from build123d import *

# Parameters (mm, degrees)
SKETCH2_W           = 63
SKETCH2_H           = 53
BOSS_EXTRUDE1_DEPTH = 121.3
BOSS_EXTRUDE2_START = 121.3
SKETCH2_3_W         = 63
SKETCH2_3_H         = 53
BOSS_EXTRUDE2_DEPTH = 28
CHAMFER5_SIZE       = 15.5
SKETCH7_R           = 6
CUT_EXTRUDE3_DEPTH  = 5.5
FILLET5_R           = 2
SHELL2_START        = 3
SHELL2_DEPTH        = 115.3
SHELL2_START_2      = 134.895176786
SHELL2_2_DEPTH      = 11.404823214
SHELL2_START_3      = 118.3
SHELL2_3_DEPTH      = 0.6
SHELL2_START_4      = -35.5
SHELL2_4_DEPTH      = 51.5
SHELL2_START_5      = 16
SHELL2_5_DEPTH      = 8.5
SHELL2_START_6      = -25.165077586
SHELL2_6_DEPTH      = 3
SKETCH4_W           = 12
SKETCH4_H           = 115.3
CUT_EXTRUDE1_DEPTH  = 175.228269807
BOSS_EXTRUDE5_START = -3
BOSS_EXTRUDE5_DEPTH = 3
CUT_EXTRUDE2_REACH  = 168.939
SKETCH6_R           = 2.1
SKETCH8_R           = 1.45
CUT_EXTRUDE4_DEPTH  = 3
BOSS_EXTRUDE6_START = 8
SKETCH8_3_R         = 1.45
BOSS_EXTRUDE6_DEPTH = 8
CUT_EXTRUDE5_REACH  = 168.939
BOSS_EXTRUDE7_START = 3
BOSS_EXTRUDE7_DEPTH = 3
CHAMFER7_SIZE       = 3
FILLET6_R           = 5


with BuildPart() as part:
    # Sketch2 → Boss-Extrude1 (new body)
    with BuildSketch(Plane(origin=(0, 0, 0), x_dir=(1, 0, 0), z_dir=(0, 1, 0))):
        Polygon((24.5, -11), (24.5, 21), (-27.6, 21), (-27.6, 4.5), (-38.5, -11), align=None)
        with Locations((-7, -37.5)):
            Rectangle(SKETCH2_W, SKETCH2_H)
    extrude(amount=BOSS_EXTRUDE1_DEPTH)

    # Sketch2<3> → Boss-Extrude2 (add)
    with BuildSketch(Plane(origin=(0, 0, 0), x_dir=(1, 0, 0), z_dir=(0, 1, 0)).offset(BOSS_EXTRUDE2_START)):
        with Locations((-7, -37.5)):
            Rectangle(SKETCH2_3_W, SKETCH2_3_H)
    extrude(amount=BOSS_EXTRUDE2_DEPTH)

    # Chamfer5
    chamfer5_edges = [part.edges().sort_by_distance(p)[0] for p in [
        (-7, 121.3, 11),
    ]]
    chamfer(chamfer5_edges, length=CHAMFER5_SIZE)

    # Sketch7 → Cut-Extrude3 (cut)
    with BuildSketch(Plane(origin=(24.5, 0, 0), x_dir=(0, 0, -1), z_dir=(1, 0, 0))):
        with Locations((-7.675, 127.9)):
            Circle(SKETCH7_R)
    extrude(amount=-CUT_EXTRUDE3_DEPTH, mode=Mode.SUBTRACT)

    # Fillet5
    fillet5_edges = [part.edges().sort_by_distance(p)[0] for p in [
        (21.75, 133.885912692, 8.085912692),
        (21.75, 127.489087308, 1.689087308),
    ]]
    fillet(fillet5_edges, radius=FILLET5_R)

    # Shell2: read off the stored shape, not the designer's step
    # Shell2 outline → Shell2 (cut)
    with BuildSketch(Plane(origin=(0, 0, 0), x_dir=(1, 0, 0), z_dir=(0, 1, 0)).offset(SHELL2_START)):
        Polygon((-24.6, 3.550767359), (-35.5, -11.949232641), (-35.5, -61), (24.5, -61), (24.5, 18), (-24.6, 18), align=None)
    extrude(amount=SHELL2_DEPTH, mode=Mode.SUBTRACT)

    # Shell2 2 outline → Shell2 2 (cut)
    with BuildSketch(Plane(origin=(0, 0, 0), x_dir=(1, 0, 0), z_dir=(0, 1, 0)).offset(SHELL2_START_2)):
        Polygon((16, -14), (-35.5, -14), (-35.5, -61), (24.5, -61), (24.5, -14), align=None)
    extrude(amount=SHELL2_2_DEPTH, mode=Mode.SUBTRACT)

    # Shell2 3 outline → Shell2 3 (cut)
    with BuildSketch(Plane(origin=(0, 0, 0), x_dir=(1, 0, 0), z_dir=(0, 1, 0)).offset(SHELL2_START_3)):
        Polygon((16, -14), (-35.5, -14), (-35.5, -61), (24.5, -61), (24.5, -14), align=None)
    extrude(amount=SHELL2_3_DEPTH, mode=Mode.SUBTRACT)

    # Shell2 4 outline → Shell2 4 (cut)
    with BuildSketch(Plane.YZ.offset(SHELL2_START_4)):
        Polygon((134.895176786, 61), (118.9, 61), (118.9, 14), (118.3, 14), (118.3, -3.257359313), (135.557359313, 14), (134.895176786, 14), align=None)
    extrude(amount=SHELL2_4_DEPTH, mode=Mode.SUBTRACT)

    # Shell2 5 outline → Shell2 5 (cut)
    with BuildSketch(Plane.YZ.offset(SHELL2_START_5)):
        with BuildLine():
            Line((134.895176786, 61), (118.9, 61))
            Line((118.9, 61), (118.9, 14))
            Line((118.9, 14), (118.3, 14))
            Line((118.3, 14), (118.3, -3.257359313))
            Line((118.3, -3.257359313), (122.237182527, 0.679823214))
            ThreePointArc((122.237182527, 0.679823214), (121.536038969, 14.038961031), (134.895176786, 13.337817473))
            Line((134.895176786, 13.337817473), (135.557359313, 14))
            Line((135.557359313, 14), (134.895176786, 14))
            Line((134.895176786, 14), (134.895176786, 61))
        make_face()
    extrude(amount=SHELL2_5_DEPTH, mode=Mode.SUBTRACT)

    # Shell2 6 outline → Shell2 6 (add)
    with BuildSketch(Plane(origin=(0, 0, 0), x_dir=(0.5752319297142107, 0, -0.8179903587679168), z_dir=(0.8179903587679168, 0, 0.5752319297142109)).offset(SHELL2_START_6)):
        Polygon((-30.1950906, 3), (-11.246212005, 3), (-11.246212005, 118.3), (-11.604905776, 118.3), (-30.1950906, 133.506591954), align=None)
    extrude(amount=SHELL2_6_DEPTH)

    # Sketch4 → Cut-Extrude1 (cut, through all)
    with BuildSketch(Plane(origin=(24.5, 0, 0), x_dir=(0, 0, -1), z_dir=(1, 0, 0))):
        with Locations((15, 60.65)):
            Rectangle(SKETCH4_W, SKETCH4_H)
    extrude(amount=-CUT_EXTRUDE1_DEPTH, mode=Mode.SUBTRACT)

    # Sketch5 → Boss-Extrude5 (add)
    with BuildSketch(Plane(origin=(24.5, 0, 0), x_dir=(0, 0, -1), z_dir=(1, 0, 0)).offset(BOSS_EXTRUDE5_START)):
        with BuildLine():
            Line((3.257359313, 118.3), (-61, 118.3))
            Line((-61, 118.3), (-61, 146.3))
            Line((-61, 146.3), (-14, 146.3))
            Line((-14, 146.3), (-14, 135.557359313))
            Line((-14, 135.557359313), (-13.337817473, 134.895176786))
            ThreePointArc((-13.337817473, 134.895176786), (-14.038961031, 121.536038969), (-0.679823214, 122.237182527))
            Line((-0.679823214, 122.237182527), (3.257359313, 118.3))
        make_face()
    extrude(amount=BOSS_EXTRUDE5_DEPTH)

    # Cut-Extrude2: up to this face of the body (flat: up to its plane)
    cut_extrude2_end = Plane(part.part.faces().sort_by_distance((-1.55, 121.3, -12.75))[0])
    # Sketch6 → Cut-Extrude2 (cut, up to the picked face)
    with BuildSketch(Plane.XZ, mode=Mode.PRIVATE) as cut_extrude2_sk1:
        with Locations(Location((-12.5, -11.5, 0), (0, 0, 270))):
            Circle(SKETCH6_R)
    cut_extrude2_tool1 = split(extrude(cut_extrude2_sk1.sketch, amount=-CUT_EXTRUDE2_REACH, mode=Mode.PRIVATE), bisect_by=cut_extrude2_end, keep=Keep.BOTH, mode=Mode.PRIVATE)
    # Sketch6 → Cut-Extrude2 (cut, up to the picked face)
    with BuildSketch(Plane.XZ, mode=Mode.PRIVATE) as cut_extrude2_sk2:
        with Locations(Location((12.5, -11.5, 0), (0, 0, 270))):
            Circle(SKETCH6_R)
    cut_extrude2_tool2 = split(extrude(cut_extrude2_sk2.sketch, amount=-CUT_EXTRUDE2_REACH, mode=Mode.PRIVATE), bisect_by=cut_extrude2_end, keep=Keep.BOTH, mode=Mode.PRIVATE)
    add(cut_extrude2_tool1.solids().sort_by(Axis((-12.5, 0, -11.5), (0, 1, 0)))[0], mode=Mode.SUBTRACT)
    add(cut_extrude2_tool2.solids().sort_by(Axis((12.5, 0, -11.5), (0, 1, 0)))[0], mode=Mode.SUBTRACT)

    # Sketch8 → Cut-Extrude4 (cut)
    with BuildSketch(Plane.XZ.offset(-146.3)):
        Polygon((17.9, 45.123529412), (11.775, 51.3), (-29.8, 51.3), (-29.8, 23.7), (11.775, 23.7), (17.9, 29.876470588), align=None)
        with Locations(Location((-7, 17.65, 0), (0, 0, 270))):
            Circle(SKETCH8_R)
        with Locations(Location((-7, 57.35, 0), (0, 0, 270))):
            Circle(SKETCH8_R)
    extrude(amount=-CUT_EXTRUDE4_DEPTH, mode=Mode.SUBTRACT)

    # Sketch8<3> → Boss-Extrude6 (add)
    # profile 1 of 2: a face of its own
    with BuildSketch(Plane.XZ.offset(-146.3).offset(BOSS_EXTRUDE6_START)):
        with BuildLine():
            Line((-12, 61), (-12, 57.35))
            ThreePointArc((-12, 57.35), (-7, 52.35), (-2, 57.35))
            Line((-2, 57.35), (-2, 61))
            Line((-2, 61), (-12, 61))
        make_face()
        with Locations(Location((-7, 57.35, 0), (0, 0, 270))):
            Circle(SKETCH8_3_R, mode=Mode.SUBTRACT)
    # profile 2 of 2: a face of its own
    with BuildSketch(Plane.XZ.offset(-146.3).offset(BOSS_EXTRUDE6_START)):
        with BuildLine():
            ThreePointArc((-2, 17.65), (-7, 22.65), (-12, 17.65))
            Line((-12, 17.65), (-12, 14))
            Line((-12, 14), (-2, 14))
            Line((-2, 14), (-2, 17.65))
        make_face()
        with Locations(Location((-7, 17.65, 0), (0, 0, 270))):
            Circle(SKETCH8_3_R, mode=Mode.SUBTRACT)
    extrude(amount=-BOSS_EXTRUDE6_DEPTH)

    # Sketch9 → Cut-Extrude5 (cut, up to next)
    with BuildSketch(Plane.XZ, mode=Mode.PRIVATE) as cut_extrude5_sk1:
        with BuildLine():
            Line((24.5, 48), (9.5, 48))
            ThreePointArc((9.5, 48), (-0.5, 38), (9.5, 28))
            Line((9.5, 28), (24.5, 28))
            Line((24.5, 28), (24.5, 48))
        make_face()
    cut_extrude5_tool1 = extrude(cut_extrude5_sk1.sketch, amount=-CUT_EXTRUDE5_REACH, mode=Mode.PRIVATE) & part.part
    add(cut_extrude5_tool1.solids().sort_by_distance((12.964021, 0, 38))[0], mode=Mode.SUBTRACT)

    # Sketch9<4> → Boss-Extrude7 (add)
    with BuildSketch(Plane.XZ.offset(BOSS_EXTRUDE7_START)):
        with BuildLine():
            ThreePointArc((9.5, 28), (-0.5, 38), (9.5, 48))
            Line((9.5, 48), (24.5, 48))
            Line((24.5, 48), (24.5, 50))
            Line((24.5, 50), (9.5, 50))
            ThreePointArc((9.5, 50), (-2.5, 38), (9.5, 26))
            Line((9.5, 26), (24.5, 26))
            Line((24.5, 26), (24.5, 28))
            Line((24.5, 28), (9.5, 28))
        make_face()
    extrude(amount=-BOSS_EXTRUDE7_DEPTH)

    # Chamfer7
    chamfer7_edges = [part.edges().sort_by_distance(p)[0] for p in [
        (17, 0, 26),
        (-2.5, 0, 38),
        (17, 0, 50),
    ]]
    chamfer(chamfer7_edges, length=CHAMFER7_SIZE - 0.0001)  # a hair under: the kernel refuses the full size

    # Fillet6
    fillet6_edges = [part.edges().sort_by_distance(p)[0] for p in [
        (-27.6, 1.5, -21),
        (24.5, 1.5, -21),
        (-27.6, 119.8, -21),
        (24.5, 119.8, -21),
    ]]
    fillet(fillet6_edges, radius=FILLET6_R)


solid = part.part
CAD build for the part. Positions are in the model's coordinates, mm. A direction names the side the tool comes from. Coordinates: 2 decimals unless noted, no trailing zeros. Loops run counter-clockwise (first coordinate to the right, second up) from the corner with the lowest first, then second, coordinate; pieces in that order, holes last. Notation, with made-up numbers: (15, -1.75) - (19, -1.75) arc R25 ccw to (19, 35.25) - close; hole circle Ø11 at (-14, 18). An arc over 180 degrees is marked (long way). Use one line per item in the form item = value. Start each with the question number.
1) Band-saw the part on C-C (y = 15.5). Give the cut face in (x, z), and give its area (3 significant figures).
2) Flat gauge pins, fed straight in: pin 1 (1.8 mm diameter, centred on x = 18.5, y = -1, fed in from +Z); pin 2 (2.5 mm diameter, centred on y = 57, z = -6.5, fed in from +X); pin 3 (4.5 mm diameter, centred on x = -7, z = 17.65, fed in from -Y); pin 4 (6.5 mm diameter, centred on x = 16, y = -1.5, fed in from -Z). Where does each tip first touch, or does it go through?
3) Band-saw the part on D-D (y = 127.9). Give the cut face in (x, z) (3 decimals), and give its area (3 significant figures).
4) Band-saw the part on A-A (x = -20). Give the cut face in (y, z).
5) Drill centre lines: L1, parallel to X at y = 119, z = -11.5; L2, parallel to Y at x = -8.5, z = 54.5; L3, parallel to Y at x = -31, z = 24.5. Where is each one in solid material? Low to high. Write a range as from..to.
6) Tool access for faces 4 (the face through (-24.6, 60, -6)), 5 (the face through (14.88, 147.78, 48.17)), 6 (the face through (-26, 60, -9)), 7 (the face through (-12, 142, 59)), 8 (the face through (-27.6, 60, -7)): list every direction of +Z, -Z, +X, -X, +Y, -Y with a clear straight run to the whole face (end or side of a thin tool).
7) Two-plate mould, pull along Y, no slides. Class faces 1 (the face through (-6, 138.3, 56)), 2 (the face through (-7.4, 129.2, 3.4)), 3 (the face through (17, -2, 51)): +Y half, -Y half, draft (parallel to the pull), parting line (faces both ways), or undercut.
Check values:
q1.outline = (-38.5, 11) - (-27.6, -4.5) - (-27.6, -9) - (-24.6, -9) - (-24.6, -3.55) - (-35.5, 11.95) - (-35.5, 61) - (24.5, 61) - (24.5, 64) - (-38.5, 64) - close
q1.area = 409 mm2
q2.pin_1 = 52.9
q2.pin_2 = -24.6
q2.pin_3 = 0
q2.pin_4 = -21
q3.outline = (-38.5, 11) - (-32.241, 2.1) - (19, 2.1) - (19, 13.675) - (24.5, 13.675) - (24.5, 64) - (-38.5, 64) - close; hole (-35.5, 11.949) - (-31.557, 6.343) - (16, 6.343) - (16, 16.675) - (21.5, 16.675) - (21.5, 61) - (-35.5, 61) - close
q3.area = 761 mm2
q4.outline = (0, -21) - (3, -21) - (3, 61) - (146.3, 61) - (146.3, 51.3) - (149.3, 51.3) - (149.3, 64) - (0, 64) - close; (118.3, -21) - (121.3, -21) - (121.3, -4.5) - (136.8, 11) - (149.3, 11) - (149.3, 23.7) - (146.3, 23.7) - (146.3, 14) - (135.56, 14) - (118.3, -3.26) - close
q5.L1 = -27.6..-14.6, -10.4..10.4, 14.6..24.5
q5.L2 = 0..3, 138.3..149.3
q5.L3 = 0..3, 146.3..149.3
q6.face_4 = -Z, +X
q6.face_5 = +Y
q6.face_6 = -Z, +X, -X
q6.face_7 = none
q6.face_8 = -Z, -X, +Y, -Y
q7.face_1 = undercut
q7.face_2 = +Y half
q7.face_3 = -Y half
